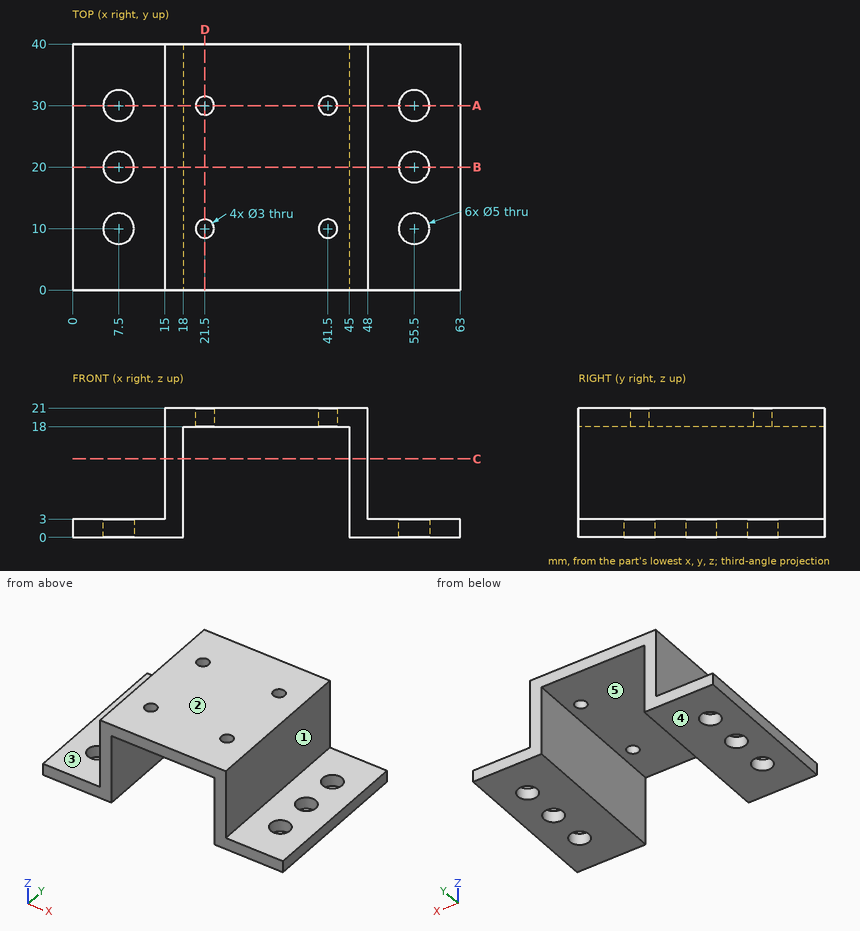
Drawing for the job (mm, zero at the part's lowest x, y, z). A direction names the side the tool comes from. Coordinates: 2 decimals unless noted, no trailing zeros. Order: outer loops, then holes, each group sorted by start corner. A loop starts at its lowest first (then second) coordinate and runs counter-clockwise, first axis right, second up. Notation, with made-up numbers: (63.25, -8.5) -> (74.25, -8.5) arc R17 cw to (74.25, 5.5) -> close; hole circle Ø10 at (53.25, 51). An arc over 180 degrees is marked (long way). One line per item, written item: value.
(1) Drop flat-ended pins along their axis: pin 1 Ø1.5 at (x, z) = (42.5, 4) entering from +Y; pin 2 Ø3 at (x, y) = (50, 5.5) entering from +Z; pin 3 Ø3.5 at (x, y) = (21.5, 30) entering from -Z. Give the stop position or say it passes through.
Checked values:
pin 1: through
pin 2: z = 3
pin 3: z = 18
(2) Slice it at B-B, the plane y = 20. List the corners of the cut face in (x, z).
Checked values:
outline: (0, 0) -> (5, 0) -> (5, 3) -> (0, 3) -> close; (10, 0) -> (18, 0) -> (18, 18) -> (45, 18) -> (45, 0) -> (53, 0) -> (53, 3) -> (48, 3) -> (48, 21) -> (15, 21) -> (15, 3) -> (10, 3) -> close; (58, 0) -> (63, 0) -> (63, 3) -> (58, 3) -> close
(3) Slice it at A-A, the plane y = 30. List the corners of the cut face in (x, z).
Checked values:
outline: (0, 0) -> (5, 0) -> (5, 3) -> (0, 3) -> close; (10, 0) -> (18, 0) -> (18, 18) -> (20, 18) -> (20, 21) -> (15, 21) -> (15, 3) -> (10, 3) -> close; (23, 18) -> (40, 18) -> (40, 21) -> (23, 21) -> close; (43, 18) -> (45, 18) -> (45, 0) -> (53, 0) -> (53, 3) -> (48, 3) -> (48, 21) -> (43, 21) -> close; (58, 0) -> (63, 0) -> (63, 3) -> (58, 3) -> close
(4) Slice it at C-C, the plane z = 12.75. List the corners of the cut face in (x, y), plus the area to 3 significant figures.
Checked values:
outline: (15, 0) -> (18, 0) -> (18, 40) -> (15, 40) -> close; (45, 0) -> (48, 0) -> (48, 40) -> (45, 40) -> close
area: 240 mm2
(5) Probe line 1 (Y direction, x = 7.5, z = 1.7); line 2 (X direction, y = 8.5, z = 8.5); line 3 (Y direction, x = 41.5, z = 18.7). List the from-to ranges inside material, lowest first. Write a range as [from, to].
Checked values:
line 1: [0, 7.5], [12.5, 17.5], [22.5, 27.5], [32.5, 40]
line 2: [15, 18], [45, 48]
line 3: [0, 8.5], [11.5, 28.5], [31.5, 40]
(6) Tool access for the marked faces 1, 2, 3, 4 and 5: list every direction of +Z, -Z, +X, -X, +Y, -Y with a clear straight run to the whole face (end or side of a thin tool).
Checked values:
face 1: +Z, +X, +Y, -Y
face 2: +Z, +X, -X, +Y, -Y
face 3: +Z, -X, +Y, -Y
face 4: -Z, +X, -X, +Y, -Y
face 5: -Z, +Y, -Y
(7) Slice it at D-D, the plane x = 21.5. List the corners of the cut face in (y, z), plus the area to 3 significant figures.
Checked values:
outline: (0, 18) -> (8.5, 18) -> (8.5, 21) -> (0, 21) -> close; (11.5, 18) -> (28.5, 18) -> (28.5, 21) -> (11.5, 21) -> close; (31.5, 18) -> (40, 18) -> (40, 21) -> (31.5, 21) -> close
area: 102 mm2
